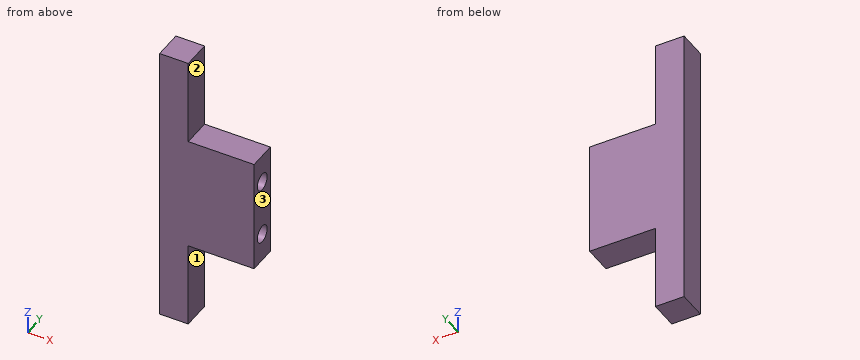
Autodesk Inventor part; units mm, degrees
ref_plane "YZ Plane" through (0, 0, 0) normal (1, 0, 0) x (0, 1, 0)
ref_plane "XZ Plane" through (0, 0, 0) normal (0, 1, 0) x (-1, 0, 0)
ref_plane "XY Plane" through (0, 0, 0) normal (0, 0, 1) x (1, 0, 0)
sketch "Esquisse1" plane through (0, 0, 0) normal (0, 1, 0) x (-1, 0, 0)
  line L0 (0, 0) -> (11.5, 0)
  line L1 (11.5, 0) -> (11.5, -20)
  line L2 (11.5, -20) -> (0, -20)
  line L3 (0, -20) -> (0, 0)
  line L4 (16.5, 15) -> (11.5, 15)
  line L5 (11.5, 15) -> (11.5, -35)
  line L6 (11.5, -35) -> (16.5, -35)
  line L7 (16.5, -35) -> (16.5, 15)
  point P0 (11.5, -10)
  dimension "d0" = 20
  dimension "d1" = 11.5
  dimension "d2" = 5
  dimension "d3" = 50
extrude "Extrusion1" add sketch "Esquisse1" along normal blind 5
sketch "Esquisse2" plane through (0, 0, 0) normal (1, 0, 0) x (0, 0, -1)
  line L0 (0, 0) -> (20, 0) construction
  line L1 (20, 0) -> (20, 5) construction
  line L2 (0, 5) -> (20, 5) construction
  line L3 (0, 0) -> (0, 5) construction
  line L4 (0, 0) -> (0, 5) construction
  line L5 (0, 2.5) -> (20, 2.5) construction
  circle A0 centre (5, 2.5) radius 1.5
  line L6 (10, 5) -> (10, 0) construction
  circle A1 centre (15, 2.5) radius 1.5
  dimension "d6" = 3
  dimension "d7" = 10
extrude "Extrusion2" cut sketch "Esquisse2" against normal blind 5
properties part number "tap_straight"
Part model, mm, in its own coordinate system. Face numbers are marked on the shaded views. A direction names the side the tool comes from. Coordinates: 2 decimals unless noted, no trailing zeros. Write each loop counter-clockwise with the first axis right and the second up, starting at its lowest first coordinate (ties: lowest second). Pieces come first, ordered by that corner, then holes. Notation, with made-up numbers: (40, 31.25) - (67, 31.25) arc R21 ccw to (67, 60.25) - close; hole circle Ø3 at (-36, 16). An arc over 180 degrees is marked (long way). Put each result on its own line as item: value.
1. Flat gauge pins, fed straight in: pin 1 Ø2.5 at (y, z) = (2.5, -28) entering from +X; pin 2 Ø1.5 at (y, z) = (2.5, -5.5) entering from +X; pin 3 Ø2.5 at (x, y) = (-4.5, 2) entering from -Z. Where does each tip first touch, or does it go through?
Final values:
pin 1: stops at x = -11.5
pin 2: stops at x = -5
pin 3: stops at z = -20
2. Band-saw the part on B-B (y = 2.5). Write the cut outline in (x, z).
Final values:
outline: (-16.5, -35) - (-11.5, -35) - (-11.5, -20) - (0, -20) - (0, -16.5) - (-5, -16.5) - (-5, -13.5) - (0, -13.5) - (0, -6.5) - (-5, -6.5) - (-5, -3.5) - (0, -3.5) - (0, 0) - (-11.5, 0) - (-11.5, 15) - (-16.5, 15) - close
3. Band-saw the part on A-A (z = -15). Write the cut outline in (x, y).
Final values:
outline: (-16.5, 0) - (0, 0) - (0, 1) - (-5, 1) - (-5, 4) - (0, 4) - (0, 5) - (-16.5, 5) - close
4. Band-saw the part on D-D (z = -22.5). Write the cut outline in (x, y), then the cut area to 3 significant figures.
Final values:
outline: (-16.5, 0) - (-11.5, 0) - (-11.5, 5) - (-16.5, 5) - close
area: 25.0 mm²
5. 3-axis set-ups, long thin cutter, end or side, ignore diameter. For the marked faces 1, 2 and 3: which of +Z, -Z, +X, -X, +Y, -Y reach the whole face in a straight line?
Final values:
face 1: -Z, +X, +Y, -Y
face 2: +Z, +X, +Y, -Y
face 3: +Z, -Z, +X, +Y, -Y
6. Band-saw the part on C-C (x = -6.5). Write the cut outline in (y, z), then the cut area to 3 significant figures.
Final values:
outline: (0, -20) - (5, -20) - (5, 0) - (0, 0) - close
area: 100 mm²
7. Probe line 1 along Y through (x, z) = (-1.6, -5); line 2 along Z through (x, y) = (-2.75, 2.9); line 3 along Z through (x, y) = (-1, 3.65). List the from-to ranges inside material, lowest first. Write a range as [from, to].
Final values:
line 1: y = [0, 1], [4, 5]
line 2: z = [-20, -16.45], [-13.55, -6.45], [-3.55, 0]
line 3: z = [-20, -15.96], [-14.04, -5.96], [-4.04, 0]
